```python
from build123d import *

# Parameters (mm, degrees)
CUT_EXTRUDE_1_DEPTH = 41
M12X1_5_1_D         = 10.5
M12X1_5_1_DEPTH     = 28.5
M12X1_5_1_TIP       = 3.15451825
CUT_EXTRUDE_2_DEPTH = 5


with BuildPart() as part:
    # 草图1 → 旋转1 (revolve)
    with BuildSketch(Plane.XY, mode=Mode.PRIVATE) as revolve_1_sk:
        Polygon((2043.973648654, 794.790077636), (2043.973648654, 776.790077638), (1926.973648645, 776.790077638), (1926.973648645, 796.790077638), (1954.473648645, 796.790077638), (1954.973648645, 796.290077638), (1954.973648645, 795.790077638), (1971.973648645, 795.790077638), (1971.973648645, 796.290077636), (1972.473648645, 796.790077636), (1987.973648648, 796.790077636), (1987.973648648, 798.790077633), (1988.47364865, 799.290077636), (1996.47364865, 799.290077636), (1996.973648654, 798.790077632), (1996.973648654, 795.790077636), (2042.973648654, 795.790077636), align=None)
    revolve(revolve_1_sk.sketch.rotate(Axis((1926.973648645, 776.790077638, 0), (1, 0, 0)), 90), axis=Axis((1926.973648645, 776.790077638, 0), (1, 0, 0)))

    # 草图5 → 切除-拉伸1 (cut)
    with BuildSketch(Plane(origin=(2043.973648654, 0, 0), x_dir=(0, 0, -1), z_dir=(1, 0, 0))):
        with BuildLine():
            Line((-8.485281368, 759.790077638), (8.485281368, 759.790077638))
            ThreePointArc((8.485281368, 759.790077638), (0, 757.790077641), (-8.485281368, 759.790077638))
        make_face()
    extrude(amount=-CUT_EXTRUDE_1_DEPTH, mode=Mode.SUBTRACT)

    # M12x1.5 螺纹孔1
    with Locations(Plane(origin=(2043.973648654, 16.946016644, 3.006019144), x_dir=(0, 0, -1), z_dir=(1, 0, 0))):
        with Locations((3.006019144, 759.844060994)):
            Hole(M12X1_5_1_D / 2, depth=M12X1_5_1_DEPTH)
            with Locations((0, 0, -(M12X1_5_1_DEPTH + M12X1_5_1_TIP / 2))):  # 118° drill point
                Cone(0, M12X1_5_1_D / 2, M12X1_5_1_TIP, mode=Mode.SUBTRACT)

    # 草图8 → 切除-拉伸2 (cut)
    with BuildSketch(Plane.XZ.offset(-759.790077638)):
        with BuildLine():
            Line((1937.973648645, 3.25), (1926.973648645, 3.25))
            Line((1926.973648645, 3.25), (1926.973648645, -3.25))
            Line((1926.973648645, -3.25), (1937.973648645, -3.25))
            ThreePointArc((1937.973648645, -3.25), (1941.223648645, 0), (1937.973648645, 3.25))
        make_face()
    extrude(amount=CUT_EXTRUDE_2_DEPTH, mode=Mode.SUBTRACT)


solid = part.part
```
Can you work these out from the model? Positions are in its coordinate system, mm. A direction names the side the tool comes from. Give positions to 0.01 mm unless a question says otherwise; leave off trailing zeros. Loops run counter-clockwise (first coordinate to the right, second up) from the corner with the lowest first, then second, coordinate; pieces in that order, holes last. Notation, with made-up numbers: M -22.75,77 L 29.25,77 A13 cw 29.25,84 Z; hole C 64,39 d10. An arc over 180 degrees is marked long. One line per question, with ' | ' between items. Start each with the question number.
Q1. If we section it at A-A (x = 2007): Please give me the cut outline in (y, z).
Q2. For pin 1 Ø8 at (x, z) = (1967, -14.5) entering from +Y; pin 2 Ø0.6 at (y, z) = (759, 2) entering from +X; pin 3 Ø0.8 at (x, y) = (1932.5, 758) entering from -Z, each with a flat end and sliding along its axis, tell me the tip position at first contact or that it passes through.
Q3. If we section it at B-B (x = 2033): Please give me the cut outline in (y, z), plus the area to 3 significant figures.
Q4. If we section it at C-C (x = 1961): Please give me the cut outline in (y, z).
Q5. For faces 1 (the flat face through (1933, 758, 3.25)), 2 (the cylindrical face through (1963.593, 763.949, -14.004)), 3 (the cylindrical face through (1940.916, 794.534, 9.229)), which set-ups out of +Z, -Z, +X, -X, +Y, -Y let a thin tool reach every point of the face, with its end or its side?
Q6. If we mould it in two halves opening along Z, with no side actions, what happens to faces 4 (the flat face through (1934, 759.79, 0)), 5 (the cylindrical face through (2020.3, 795.34, -4.12)), 6 (the flat face through (1996.974, 758.8, -6.6))? For each: +Z half, -Z half, draft (parallel to the pull), parting line (faces both ways), or undercut.
Q7. If I drill on line 1 (Y direction, x = 2032, z = 0); line 2 (X direction, y = 786, z = 20); line 3 (X direction, y = 776.5, z = -18), over which ranges is the centre line in solid material (lowest first)? Write a range as from..to.
Computed:
1) outline: M 759.79,-8.49 A19 ccw long 759.79,8.49 Z
2) pin 1: stops at y = 792.63 | pin 2: stops at x = 2002.97 | pin 3: stops at z = -7.86
3) outline: M 759.79,-8.49 A19 ccw long 759.79,8.49 Z; hole C 776.79,0 d10.5 | area: 1,020 mm²
4) outline: C 776.79,0 d38
5) face 1: -X, -Y | face 2: none | face 3: -X
6) face 4: undercut | face 5: parting line | face 6: draft
7) line 1: y = 759.79..771.54, 782.04..795.79 | line 2: x = 1987.99..1996.95 | line 3: x = 1926.97..2043.97
